from build123d import *

# Parameters (mm, degrees)
SKETCH1_R           = 6.35
BOSS_EXTRUDE1_DEPTH = 18.542
CUT_EXTRUDE1_DEPTH  = 92.872891976


with BuildPart() as part:
    # Sketch1 → Boss-Extrude1 (new, symmetric)
    with BuildSketch(Plane.XY):
        with BuildLine():
            Line((-63.5, -33.274), (63.5, -33.274))
            Line((63.5, -33.274), (63.5, -19.304))
            Line((63.5, -19.304), (31.75, -19.304))
            Line((31.75, -19.304), (31.75, -1.27))
            ThreePointArc((31.75, -1.27), (0, 30.48), (-31.75, -1.27))
            Line((-31.75, -1.27), (-31.75, -19.304))
            Line((-31.75, -19.304), (-63.5, -19.304))
            Line((-63.5, -19.304), (-63.5, -33.274))
        make_face()
        Circle(SKETCH1_R, mode=Mode.SUBTRACT)
    extrude(amount=BOSS_EXTRUDE1_DEPTH, both=True)

    # Sketch2 → Cut-Extrude1 (cut, through all)
    with BuildSketch(Plane.XZ.offset(33.274)):
        with BuildLine():
            Line((-49.53, 6.477), (-46.482, 6.477))
            ThreePointArc((-46.482, 6.477), (-40.005, 0), (-46.482, -6.477))
            Line((-46.482, -6.477), (-49.53, -6.477))
            ThreePointArc((-49.53, -6.477), (-56.007, 0), (-49.53, 6.477))
        make_face()
        with BuildLine():
            Line((49.53, 6.477), (46.482, 6.477))
            ThreePointArc((46.482, 6.477), (40.005, 0), (46.482, -6.477))
            Line((46.482, -6.477), (49.53, -6.477))
            ThreePointArc((49.53, -6.477), (56.007, 0), (49.53, 6.477))
        make_face()
    extrude(amount=-CUT_EXTRUDE1_DEPTH, mode=Mode.SUBTRACT)


solid = part.part
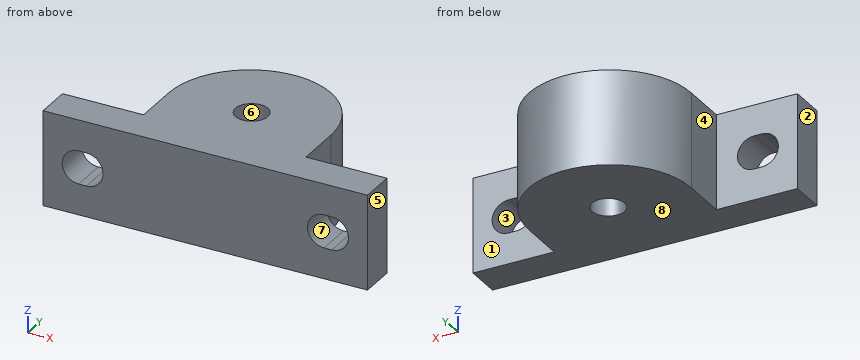
The listing builds one solid part. Answer for the finished solid, in the listing's coordinates (mm). Face numbers are marked on the shaded views. A direction names the side the tool comes from. Give positions to 0.01 mm unless a question says otherwise; leave off trailing zeros. Order: outer loops, then holes, each group sorted by start corner. A loop starts at its lowest first (then second) coordinate and runs counter-clockwise, first axis right, second up. Notation, with made-up numbers: (11, 64.25) - (17, 64.25) arc R7 cw to (17, 69.25) - close; hole circle Ø8 at (35, 38). An arc over 180 degrees is marked (long way). One line per item, written item: value. Start each with the question number.
1) A cutting plane is placed at D-D on z = 15. Give the vertices of the cut face in (x, y), then the cut area to 3 significant figures.
2) A cutting plane is placed at A-A on z = 0. Give the vertices of the cut face in (x, y) (3 decimals).
3) A cutting plane is placed at C-C on y = 0. Give the vertices of the cut face in (x, z), then the cut area to 3 significant figures.
4) Find the intervals of material crossed by L1, parallel to Y at x = 0, z = 11; L2, parallel to Y at x = -36, z = -4; L3, parallel to X at y = -9, z = -13.5, in increasing order.
5) The mould has two halves that part along Z. Classify the marked faces 6, 7 and 8: released by +Z, released by -Z, zero draft, split by the parting line, or undercut.
6) A tool of negligible diameter and unlimited length cuts with its end or side. For the marked faces 1, 2, 3, 4 and 5, from which of +Z, -Z, +X, -X, +Y, -Y can it reach the whole face along a straight path? Write none if from no direction.
7) A cutting plane is placed at B-B on x = 0. Give the vertices of the cut face in (y, z).
8) Given pin 1 Ø1 at (y, z) = (22.5, -6) entering from -X; pin 2 Ø6 at (y, z) = (11, -7) entering from -X; pin 3 Ø9.5 at (x, z) = (-48.5, -8) entering from +Y, each flat-ended and moving along its own axis, determine where each tip first touches the part or whether it passes through.
Answer sheet:
1. outline: (-63.5, -33.27) - (63.5, -33.27) - (63.5, -19.3) - (31.75, -19.3) - (31.75, -1.27) arc R31.75 ccw to (-31.75, -1.27) - (-31.75, -19.3) - (-63.5, -19.3) - close; hole circle Ø12.7 at (0, 0)
1. area: 4,380 mm2
2. outline: (-63.5, -33.274) - (-56.007, -33.274) - (-56.007, -19.304) - (-63.5, -19.304) - close; (-40.005, -33.274) - (40.005, -33.274) - (40.005, -19.304) - (31.75, -19.304) - (31.75, -1.27) arc R31.75 ccw to (-31.75, -1.27) - (-31.75, -19.304) - (-40.005, -19.304) - close; (56.007, -33.274) - (63.5, -33.274) - (63.5, -19.304) - (56.007, -19.304) - close; hole circle Ø12.7 at (0, 0)
3. outline: (-31.72, -18.54) - (-6.35, -18.54) - (-6.35, 18.54) - (-31.72, 18.54) - close; (6.35, -18.54) - (31.72, -18.54) - (31.72, 18.54) - (6.35, 18.54) - close
3. area: 1,880 mm2
4. L1: y = -33.27 to -6.35, 6.35 to 30.48
4. L2: y = -33.27 to -19.3
4. L3: x = -31.75 to 31.75
5. face 6: zero draft
5. face 7: undercut
5. face 8: released by -Z
6. face 1: +Z, -Z, +X, +Y
6. face 2: +Z, -Z, -X, +Y, -Y
6. face 3: +Y, -Y
6. face 4: +Z, -Z, -X, +Y
6. face 5: +Z, -Z, +X, +Y, -Y
7. outline: (-33.27, -18.54) - (-6.35, -18.54) - (-6.35, 18.54) - (-33.27, 18.54) - close; (6.35, -18.54) - (30.48, -18.54) - (30.48, 18.54) - (6.35, 18.54) - close
8. pin 1: stops at x = -21.6
8. pin 2: stops at x = -30.37
8. pin 3: stops at y = -19.3
